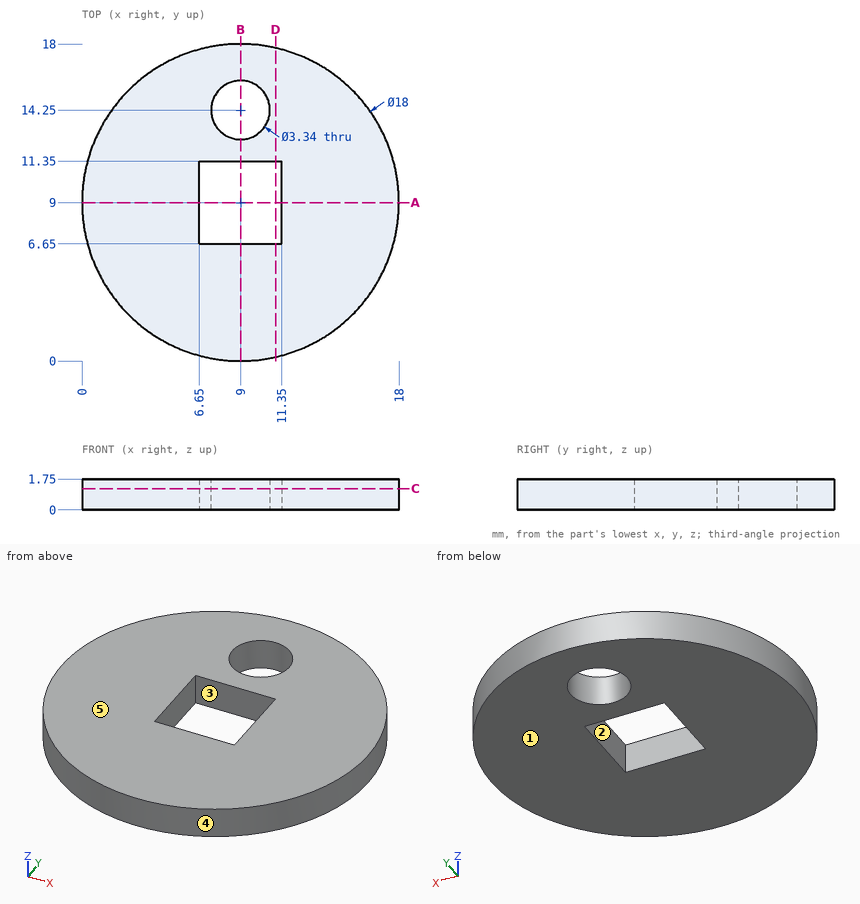
Geometry: see drawing. Coordinates: mm, zero at the bounding-box minimum. A direction names the side the tool comes from. Give positions to 0.01 mm unless a question says otherwise; leave off trailing zeros. Loops run counter-clockwise (first coordinate to the right, second up) from the corner with the lowest first, then second, coordinate; pieces in that order, holes last. Notation, with made-up numbers: (-23, -11.5) -> (36, -11.5) arc R16 ccw to (36, 0.5) -> close; hole circle Ø9 at (16, 6.25). An arc over 180 degrees is marked (long way). Answer as a JSON object with one key per item and string values. Group by question number.
Item 1: Cut plane D-D, the plane x = 11. Return the cut outline in (y, z), and give its area (3 significant figures).
Item 2: Reachability of the marked faces 1 and 2 from +Z, -Z, +X, -X, +Y, -Y: full face, straight path, thin tool, end or side. Return the list, or none.
Item 3: Cut plane A-A, the plane y = 9. Return the cut outline in (x, z).
Item 4: Cut plane C-C, the plane z = 1.2. Return the cut outline in (x, y), and give its area (3 significant figures).
Item 5: Cut plane B-B, the plane x = 9. Return the cut outline in (y, z).
Item 6: Line query: probe 1 along Y at (x, z) = (9, 1.4); probe 2 along X at (y, z) = (9.75, 1.6); probe 3 along X at (y, z) = (13.75, 0.55). Output: solid intervals per line, ascending.
Item 7: Pull-direction query (X, two-part tool) for the marked faces 3, 4 and 5; classes: released by +X, released by -X, zero draft, split by the parting line, or undercut.
Item 8: Pin query (flat end, axial travel): P1, Ø2.5, axis at x = 9, y = 14.25, coming from the -Z side. Return the tip coordinate at first contact, or that it passes through.
Checks:
{
 "1": {"outline": "(0.23, 0) -> (6.65, 0) -> (6.65, 1.75) -> (0.23, 1.75) -> close; (11.35, 0) -> (17.77, 0) -> (17.77, 1.75) -> (11.35, 1.75) -> close", "area": "22.5 mm²"},
 "2": {"face 1": "-Z, +X, -X, +Y, -Y", "face 2": "+Z, -Z"},
 "3": {"outline": "(0, 0) -> (6.65, 0) -> (6.65, 1.75) -> (0, 1.75) -> close; (11.35, 0) -> (18, 0) -> (18, 1.75) -> (11.35, 1.75) -> close"},
 "4": {"outline": "circle Ø18 at (9, 9); hole (6.65, 6.65) -> (11.35, 6.65) -> (11.35, 11.35) -> (6.65, 11.35) -> close; hole circle Ø3.34 at (9, 14.25)", "area": "224 mm²"},
 "5": {"outline": "(0, 0) -> (6.65, 0) -> (6.65, 1.75) -> (0, 1.75) -> close; (11.35, 0) -> (12.58, 0) -> (12.58, 1.75) -> (11.35, 1.75) -> close; (15.92, 0) -> (18, 0) -> (18, 1.75) -> (15.92, 1.75) -> close"},
 "6": {"probe 1": "y = 0 to 6.65, 11.35 to 12.58, 15.92 to 18", "probe 2": "x = 0.03 to 6.65, 11.35 to 17.97", "probe 3": "x = 1.36 to 7.41, 10.59 to 16.64"},
 "7": {"face 3": "undercut", "face 4": "split by the parting line", "face 5": "zero draft"},
 "8": {"P1": "passes through"}
}
